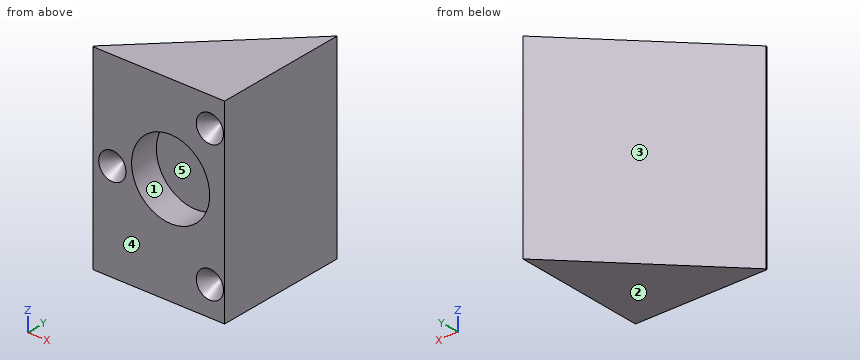
Autodesk Inventor part; units mm, degrees
ref_plane "YZ Plane" through (0, 0, 0) normal (1, 0, 0) x (0, 1, 0)
ref_plane "XZ Plane" through (0, 0, 0) normal (0, 1, 0) x (-1, 0, 0)
ref_plane "XY Plane" through (0, 0, 0) normal (0, 0, 1) x (1, 0, 0)
ref_plane "Arbeitsebene1" through (0, 0, 1) normal (0, 0, 1) x (1, 0, 0)
sketch "Skizze1" plane through (0, 0, 1) normal (0, 0, 1) x (1, 0, 0)
  line L0 (0, -25) -> (0, 0)
  line L1 (0, -25) -> (14, -25)
  line L2 (14, 0) -> (14, -25)
  line L3 (0, 0) -> (14, 0)
  line L4 (-1, -11.3514) -> (-6.5, -11.3514) construction
  line L5 (-4.5, -14.125) -> (-37.3, -14.125) construction
  line L6 (-1, -16.6486) -> (-6.5, -16.6486) construction
  line L7 (4, 20.8392) -> (4, 0) construction
  line L8 (12, 20.8392) -> (12, 0) construction
  line L9 (8, 20.6561) -> (8, -14) construction
  line L10 (-4.5, -14) -> (8, -14) construction
  line L11 (1.6137, -20.3863) -> (12.8954, -9.1046) construction
  line L12 (1.6137, -20.3863) -> (17.5684, -20.3863) construction
  line L13 (0, -25) -> (14, -25) construction
  line L14 (0, -24.6915) -> (13.5, -24.6915)
  line L15 (13.5, -24.6915) -> (13.5, -11.0456)
  line L16 (13.5, -11.0456) -> (0, -24.5456)
  line L17 (0, -24.6915) -> (0, -24.5456)
  dimension "d0" = 4
  dimension "d1" = 5.2972
  dimension "d2" = 2.6486
  dimension "d3" = 45
  dimension "d4" = 1.8
  dimension "d5" = 0.5
extrude "Extrusion1" add sketch "Skizze1" along normal blind 20 contours L0 L16 L15 L14
sketch "Skizze2" plane through (0, -24.6915, 1) normal (0, -1, 0) x (1, 0, 0)
  circle A0 centre (12, 17) radius 1.4
  line L0 (0, 2.559) -> (10.6713, 2.559)
  circle A1 centre (12, 3) radius 1.4
  circle A2 centre (2, 10) radius 1.4
  point P0 (0, -1)
hole "Bohrung1" at (12, -24.6915, 18) at (12, -24.6915, 4) at (2, -24.6915, 11) direction (0, 1, 0) diameter 2.8 depth 0.001 tip angle 80
sketch "Skizze3" plane through (0, -24.6915, 1) normal (0, -1, 0) x (1, 0, 0)
  line L0 (0, 20) -> (13.5, 20)
  line L1 (0, 0) -> (13.5, 0)
  line L2 (13.5, 0) -> (13.5, 20)
  line L3 (0, -7) -> (0, 29)
  circle A0 centre (7.9714, 11) radius 4
  point P0 (0, -1)
  dimension "d15" = 8
extrude "Extrusion2" cut sketch "Skizze3" against normal blind 3 contours A0
equation "\"d2\" = 0.5 * d1"
properties part number "TIRFImager_KinematicMirror_v3"
Verification items for the finished model (mm, model axes). Face numbers are marked on the shaded views. A direction names the side the tool comes from. Give positions to 0.01 mm unless a question says otherwise; leave off trailing zeros. Write each loop counter-clockwise with the first axis right and the second up, starting at its lowest first coordinate (ties: lowest second). Pieces come first, ordered by that corner, then holes.
(1) Access from +Z, -Z, +X, -X, +Y, -Y to the whole of each face (thin tool, end or side, straight path). Record for the marked faces 4 and 5.
(2) Mould release check, pull along X, two halves, no side actions. Record for the marked faces 1, 2 and 3: +X half, -X half, draft (parallel to the pull), parting line (faces both ways), or undercut.
(3) Cross-section at C-C (y = -16.5). Enter the section's corners in (x, z), plus the area to 3 significant figures.
(4) Material ranges on line 1 (X direction, y = -23.5, z = 14.25); line 2 (Z direction, x = 5.5, y = -23); line 3 (X direction, y = -14.25, z = 15.5), recorded low to high.
(5) Cross-section at B-B (z = 6). Enter the section's corners in (x, y).
(6) Cross-section at A-A (x = 8.75). Enter the section's corners in (y, z), plus the area to 3 significant figures.
(7) Cross-section at D-D (x = 4.25). Enter the section's corners in (y, z).
(8) Gauge pin test, flat ends, axial feed: pin 1 (1.5 mm diameter, centred on x = 10, z = 7.5, fed in from +Y); pin 2 (8 mm diameter, centred on x = 2.5, z = 4.5, fed in from +Y); pin 3 (4.5 mm diameter, centred on x = 2, z = 11, fed in from +Y). Record the tip position at first contact, or that the pin passes through.
Worked out:
1. face 4: +Z, -Z, +X, -X, -Y
1. face 5: -Y
2. face 1: undercut
2. face 2: draft
2. face 3: -X half
3. outline: (8.05, 1) - (13.5, 1) - (13.5, 21) - (8.05, 21) - close
3. area: 109 mm2
4. line 1: x = 1.05 to 4.66, 11.28 to 13.5
4. line 2: z = 1 to 8.85, 15.15 to 21
4. line 3: x = 10.3 to 13.5
5. outline: (0, -24.69) - (13.5, -24.69) - (13.5, -11.05) - (0, -24.55) - close
6. outline: (-24.69, 1) - (-15.8, 1) - (-15.8, 21) - (-24.69, 21) - (-24.69, 15.92) - (-21.69, 15.92) - (-21.69, 8.08) - (-24.69, 8.08) - close
6. area: 154 mm2
7. outline: (-24.69, 1) - (-20.3, 1) - (-20.3, 21) - (-24.69, 21) - (-24.69, 13.47) - (-21.69, 13.47) - (-21.69, 10.53) - (-24.69, 10.53) - close
8. pin 1: stops at y = -13.8
8. pin 2: stops at y = -18.05
8. pin 3: stops at y = -20.3
